```python
from build123d import *

# Parameters (mm, degrees)
SKETCH1_R           = 1.5
BOSS_EXTRUDE1_DEPTH = 5.72


with BuildPart() as part:
    # Sketch1 → Boss-Extrude1 (new body)
    with BuildSketch(Plane.XY):
        with BuildLine():
            Line((0, 0), (10, 0))
            Line((10, 0), (10, -9.381049961))
            ThreePointArc((10, -9.381049961), (5, -21), (10, -32.618950039))
            Line((10, -32.618950039), (10, -42))
            Line((10, -42), (0, -42))
            Line((0, -42), (0, 0))
        make_face()
        with Locations((5.5, -38)):
            Circle(SKETCH1_R, mode=Mode.SUBTRACT)
        with Locations((5.5, -4)):
            Circle(SKETCH1_R, mode=Mode.SUBTRACT)
    extrude(amount=BOSS_EXTRUDE1_DEPTH)


solid = part.part
```
Could you check a few things on this model? Use its own coordinates, in mm. Give positions to 0.01 mm unless a question says otherwise; leave off trailing zeros. Loops run counter-clockwise (first coordinate to the right, second up) from the corner with the lowest first, then second, coordinate; pieces in that order, holes last. Notation, with made-up numbers: (-38.75, -14.75) - (16.25, -14.75) arc R22 cw to (16.25, -5.75) - close; hole circle Ø8 at (36, 33.5). An arc over 180 degrees is marked (long way). Answer in a Markdown table with one row per item. Add a question column.
Q1. If we section it at B-B (y = -4): List the corners of the cut face in (x, z) for me.
Q2. If we section it at C-C (x = 8): List the corners of the cut face in (y, z) for me.
Q3. If we section it at A-A (z = 0.55): List the corners of the cut face in (x, y) for me.
Q4. For pin 1 (1.8 mm diameter, centred on x = 5.5, y = -38, fed in from +Z); pin 2 (1 mm diameter, centred on y = -31, z = 2.5, fed in from +X); pin 3 (1 mm diameter, centred on y = -12.5, z = 3, fed in from +X), each with a flat end and sliding along its axis, tell me the tip position at first contact or that it passes through.
Q5. Please list where these lines run through material, in increasing order: L1, parallel to Y at x = 6.5, z = 3.1; L2, parallel to X at y = -37.5, z = 1.05; L3, parallel to X at y = -17, z = 1.6. Write a range as from..to.
Q6. We'd pull the mould along X, two halves only. Please class faces 1 (the face through (4, -21, 0)), 2 (the face through (4.39, -2.99, 2.82)), 3 (the face through (10, -5, 3)): +X half, -X half, draft (parallel to the pull), parting line (faces both ways), or undercut.
Q7. If we section it at D-D (x = 5.5): List the corners of the cut face in (y, z) for me, plus the area to 3 significant figures.
The answers:
| question | item | result |
|---|---|---|
| 1 | outline | (0, 0) - (4, 0) - (4, 5.72) - (0, 5.72) - close; (7, 0) - (10, 0) - (10, 5.72) - (7, 5.72) - close |
| 2 | outline | (-42, 0) - (-30.33, 0) - (-30.33, 5.72) - (-42, 5.72) - close; (-11.67, 0) - (0, 0) - (0, 5.72) - (-11.67, 5.72) - close |
| 3 | outline | (0, -42) - (10, -42) - (10, -32.62) arc R16 cw to (10, -9.38) - (10, 0) - (0, 0) - close; hole circle Ø3 at (5.5, -38); hole circle Ø3 at (5.5, -4) |
| 4 | pin 1 | passes through |
| 4 | pin 2 | stops at x = 8.93 |
| 4 | pin 3 | stops at x = 7.77 |
| 5 | L1 | y = -42..-39.12, -36.88..-27.76, -14.24..-5.12, -2.88..0 |
| 5 | L2 | x = 0..4.09, 6.91..10 |
| 5 | L3 | x = 0..5.51 |
| 6 | face 1 | draft |
| 6 | face 2 | undercut |
| 6 | face 3 | +X half |
| 7 | outline | (-42, 0) - (-39.5, 0) - (-39.5, 5.72) - (-42, 5.72) - close; (-36.5, 0) - (-24.97, 0) - (-24.97, 5.72) - (-36.5, 5.72) - close; (-17.03, 0) - (-5.5, 0) - (-5.5, 5.72) - (-17.03, 5.72) - close; (-2.5, 0) - (0, 0) - (0, 5.72) - (-2.5, 5.72) - close |
| 7 | area | 161 mm^2 |
